Autodesk Inventor part; units mm, degrees
ref_plane "YZ Plane" through (0, 0, 0) normal (1, 0, 0) x (0, 1, 0)
ref_plane "XZ Plane" through (0, 0, 0) normal (0, 1, 0) x (-1, 0, 0)
ref_plane "XY Plane" through (0, 0, 0) normal (0, 0, 1) x (1, 0, 0)
sketch "Sketch1" plane through (0, 0, 0) normal (0, 0, 1) x (1, 0, 0)
  line L0 (9.7809, 25.2857) -> (14.7809, 25.2857)
  line L1 (14.7809, 25.2857) -> (14.7809, 5.2857)
  line L2 (14.7809, 5.2857) -> (9.7809, 5.2857)
  line L3 (9.7809, 5.2857) -> (9.7809, 25.2857)
  line L4 (14.7809, 35.2857) -> (44.7809, 35.2857)
  line L5 (44.7809, 35.2857) -> (44.7809, -4.7143)
  line L6 (44.7809, -4.7143) -> (14.7809, -4.7143)
  line L7 (14.7809, -4.7143) -> (14.7809, 35.2857)
  circle A0 centre (29.7809, 15.2857) radius 3.5
  point P0 (0, 0)
  point P1 (12.2809, 25.2857)
  dimension "d0" = 5
  dimension "d1" = 20
  dimension "d2" = 30
  dimension "d3" = 40
  dimension "d4" = 10
  dimension "d7" = 7
extrude "Extrusion1" add sketch "Sketch1" along normal blind 5 contours L0 L1 L2 L3 | L7 L4 L5 L6 L1 | A0
extrude "Extrusion2" cut sketch "Sketch1" along normal blind 5 contours A0
Design review of the part built by this model. Coordinates are the model's own, in mm. A direction names the side the tool comes from. Coordinates: 2 decimals unless noted, no trailing zeros. Write each loop counter-clockwise with the first axis right and the second up, starting at its lowest first coordinate (ties: lowest second). Pieces come first, ordered by that corner, then holes. Notation, with made-up numbers: M 0.5,79 L 17.5,79 A26 ccw 17.5,94 Z; hole C -18,48 d5. An arc over 180 degrees is marked long. Answer as a JSON object with one key per item and string values.
Item 1: Add section B-B, the plane z = 3.8. Give the boundary of the cut face in (x, y).
Outcome:
{"outline": "M 9.78,5.29 L 14.78,5.29 L 14.78,-4.71 L 44.78,-4.71 L 44.78,35.29 L 14.78,35.29 L 14.78,25.29 L 9.78,25.29 Z; hole C 29.78,15.29 d7"}
Item 2: Add section A-A, the plane y = 17.5. Give the boundary of the cut face in (x, z), and give its area (3 significant figures).
Outcome:
{"outline": "M 9.78,0 L 27.07,0 L 27.07,5 L 9.78,5 Z; M 32.49,0 L 44.78,0 L 44.78,5 L 32.49,5 Z", "area": "148 mm²"}
Item 3: Machinability: for faces 1 (the flat face through (12, 25.286, 2)), 2 (the flat face through (12, 5.286, 2)), 3 (the flat face through (44.781, 16, 2)), which of the approach directions +Z, -Z, +X, -X, +Y, -Y give a long, thin tool a straight path to every point of the face, cutting with its end or side? Answer none if there is none.
Outcome:
{"face 1": "+Z, -Z, -X, +Y", "face 2": "+Z, -Z, -X, -Y", "face 3": "+Z, -Z, +X, +Y, -Y"}
Item 4: Draft analysis for pull direction X (two halves, no side actions). For faces 4 (the cylindrical face through (26.284, 15.132, 2.465)), 5 (the flat face through (27, 20, 5)), 6 (the flat face through (9.781, 15, 2)), state which applies: pulls with the +X half, pulls with the -X half, needs draft (parallel to the pull), parting line crosses it, or undercut.
Outcome:
{"face 4": "undercut", "face 5": "needs draft", "face 6": "pulls with the -X half"}
Item 5: Add section C-C, the plane x = 13.5. Give the boundary of the cut face in (y, z).
Outcome:
{"outline": "M 5.29,0 L 25.29,0 L 25.29,5 L 5.29,5 Z"}
Item 6: Add section D-D, the plane y = 0.5. Give the boundary of the cut face in (x, z).
Outcome:
{"outline": "M 14.78,0 L 44.78,0 L 44.78,5 L 14.78,5 Z"}
Item 7: Insertion check: pin 1 Ø2.5 at (x, z) = (11, 2) entering from -Y; pin 2 Ø8 at (x, y) = (29.78, 15.29) entering from +Z; pin 3 Ø1.5 at (y, z) = (31, 3) entering from -X; pin 4 Ø1.5 at (x, z) = (12, 3) entering from +Y. Each pin has a flat end and moves straight along its axis. Give the tip position at first contact, or say it passes through.
Outcome:
{"pin 1": "y = 5.29", "pin 2": "z = 5", "pin 3": "x = 14.78", "pin 4": "y = 25.29"}
Item 8: Wall thickness on probe 1 along X at (y, z) = (15.5, 0.6); probe 2 along X at (y, z) = (0, 3.45); probe 3 along X at (y, z) = (16, 4.05): over which ranges is each line inside the solid? List them lowest first.
Outcome:
{"probe 1": "9.78 to 26.29, 33.27 to 44.78", "probe 2": "14.78 to 44.78", "probe 3": "9.78 to 26.35, 33.21 to 44.78"}
